```python
from build123d import *

# Parameters (mm, degrees)
F0_W          = 11.8681662488
F0_H          = 19.05
F1_DEPTH      = 12.7
F1_DEPTH_BACK = 12.7
F2_DEPTH      = 6.35
F2_DEPTH_BACK = 6.35
F3_DEPTH      = 12.7
F3_DEPTH_BACK = 12.7
F0_H_2        = 6.35
F4_DEPTH      = 12.7
F4_DEPTH_BACK = 12.7
F6_DEPTH      = 12.7


with BuildPart() as f1:
    # F0 (on Front) → F1 (new body, two sides)
    with BuildSketch(Plane.XZ) as f1_sk:
        with Locations((-36.0392803956, -20.5900701019)):
            Rectangle(F0_W, F0_H)
    extrude(amount=F1_DEPTH)
    extrude(f1_sk.sketch, amount=-F1_DEPTH_BACK)

    # F0 (on Front) → F2 (join, two sides)
    with BuildSketch(Plane.XZ) as f2_sk:
        with BuildLine():
            Line((-30.1051972712, -11.0650701019), (-30.1051972712, -30.1150701019))
            Line((-30.1051972712, -30.1150701019), (-16.57336352, -30.1150701019))
            ThreePointArc((-16.57336352, -30.1150701019), (-26.09836352, -20.5900701019), (-16.57336352, -11.0650701019))
            Line((-16.57336352, -11.0650701019), (-30.1051972712, -11.0650701019))
        make_face()
    extrude(amount=F2_DEPTH)
    extrude(f2_sk.sketch, amount=-F2_DEPTH_BACK)

    # F0 (on Front) → F3 (join, two sides)
    with BuildSketch(Plane.XZ) as f3_sk:
        with BuildLine():
            Line((-16.57336352, -26.9400701019), (-16.57336352, -30.1150701019))
            ThreePointArc((-16.57336352, -30.1150701019), (-9.8381714292, -27.3252621927), (-7.04836352, -20.5900701019))
            ThreePointArc((-7.04836352, -20.5900701019), (-9.8381714292, -13.8548780111), (-16.57336352, -11.0650701019))
            Line((-16.57336352, -11.0650701019), (-16.57336352, -14.2400701019))
            ThreePointArc((-16.57336352, -14.2400701019), (-12.0832354595, -16.0999420414), (-10.22336352, -20.5900701019))
            ThreePointArc((-10.22336352, -20.5900701019), (-12.0832354595, -25.0801981625), (-16.57336352, -26.9400701019))
        make_face()
        with BuildLine():
            ThreePointArc((-16.57336352, -11.0650701019), (-26.09836352, -20.5900701019), (-16.57336352, -30.1150701019))
            Line((-16.57336352, -30.1150701019), (-16.57336352, -26.9400701019))
            ThreePointArc((-16.57336352, -26.9400701019), (-22.92336352, -20.5900701019), (-16.57336352, -14.2400701019))
            Line((-16.57336352, -14.2400701019), (-16.57336352, -11.0650701019))
        make_face()
    extrude(amount=F3_DEPTH)
    extrude(f3_sk.sketch, amount=-F3_DEPTH_BACK)

    # F0 (on Front) → F4 (join, two sides)
    with BuildSketch(Plane.XZ) as f4_sk:
        with Locations((-36.0392803956, -7.8900701019)):
            Rectangle(F0_W, F0_H_2)
    extrude(amount=F4_DEPTH)
    extrude(f4_sk.sketch, amount=-F4_DEPTH_BACK)

    # F5 (on face) → F6 (cut)
    with BuildSketch(Plane.YZ.offset(-30.1051972712)):
        Polygon((12.7, -4.7150701019), (6.35, -4.7150701019), (12.7, -11.0650701019), align=None)
        Polygon((-12.7, -11.0650701019), (-6.35, -4.7150701019), (-12.7, -4.7150701019), align=None)
    extrude(amount=-F6_DEPTH, mode=Mode.SUBTRACT)


solid = f1.part
```
Check sheet for the modelled part. Datum: model origin and axes. Units: mm. A direction names the side the tool comes from. Round coordinates to 2 decimals unless told otherwise and drop trailing zeros. Loops run counter-clockwise (first coordinate to the right, second up) from the corner with the lowest first, then second, coordinate; pieces in that order, holes last. Notation, with made-up numbers: (2, -3.75) -> (41, -3.75) arc R33 ccw to (41, 28.25) -> close; hole circle Ø2 at (57, 4). An arc over 180 degrees is marked (long way). Write item = value, one per line. Start each with the question number.
1) Thickness scan on probe 1 along X at (y, z) = (-10.25, -13.5); probe 2 along X at (y, z) = (-7, -15); probe 3 along Z at (x, y) = (-25, 0.5). Record the ranges inside material, lowest first.
2) Release check for a two-part mould opening along X. For faces 1 (the flat face through (-26.4, 6.35, -20.5)), 2 (the flat face through (-41.973, 0, -18)), 3 (the flat face through (-36, -12.7, -20)) record: released by +X, released by -X, zero draft, split by the parting line, or undercut.
3) Gauge pin test, flat ends, axial feed: pin 1 Ø5 at (y, z) = (2.5, -8.5) entering from +X; pin 2 Ø1.5 at (x, y) = (-12.5, 6.5) entering from -Z; pin 3 Ø5 at (x, z) = (-38, -7.5) entering from +Y. Record the tip position at first contact, or that the pin passes through.
4) Sectioned sample at A-A, the plane y = -8. Record the cut outline in (x, z) (3 decimals).
5) Sectioned sample at B-B, the plane x = -19.5. Record the cut outline in (y, z).
6) Sectioned sample at C-C, the plane y = 2.25. Record the cut outline in (x, z) (3 decimals), plus the area to 3 significant figures.
7) Sectioned sample at D-D, the plane z = -28.5. Record the cut outline in (x, y), plus the area to 3 significant figures.
8) Set-up check for faces 4 (the flat face through (-36, 12.7, -20)), 5 (the flat face through (-23, 0, -11.065)), 6 (the flat face through (-30.105, 0, -9)): record each of +Z, -Z, +X, -X, +Y, -Y from which the full face is reachable in a straight line by a thin tool's end or side.
Results are:
q1.probe_1 = -41.97 to -30.11, -22.93 to -10.21
q1.probe_2 = -41.97 to -30.11, -24.29 to -19.59, -13.56 to -8.86
q1.probe_3 = -30.12 to -11.07
q2.face_1 = undercut
q2.face_2 = released by -X
q2.face_3 = zero draft
q3.pin_1 = -30.11
q3.pin_2 = -29.52
q3.pin_3 = 11.63
q4.outline = (-41.973, -30.115) -> (-30.105, -30.115) -> (-30.105, -6.365) -> (-41.973, -6.365) -> close; circle Ø19.05 at (-16.573, -20.59); hole circle Ø12.7 at (-16.573, -20.59)
q5.outline = (-12.7, -29.65) -> (-6.35, -29.65) -> (-6.35, -30.12) -> (6.35, -30.12) -> (6.35, -29.65) -> (12.7, -29.65) -> (12.7, -26.23) -> (-12.7, -26.23) -> close; (-12.7, -14.95) -> (12.7, -14.95) -> (12.7, -11.53) -> (6.35, -11.53) -> (6.35, -11.07) -> (-6.35, -11.07) -> (-6.35, -11.53) -> (-12.7, -11.53) -> close
q6.outline = (-41.973, -30.115) -> (-16.573, -30.115) arc R9.525 ccw to (-16.573, -11.065) -> (-30.105, -11.065) -> (-30.105, -4.715) -> (-41.973, -4.715) -> close; hole circle Ø12.7 at (-16.573, -20.59)
q6.area = 575 mm^2
q7.outline = (-41.97, -12.7) -> (-30.11, -12.7) -> (-30.11, -6.35) -> (-21.88, -6.35) -> (-21.88, -12.7) -> (-11.27, -12.7) -> (-11.27, 12.7) -> (-21.88, 12.7) -> (-21.88, 6.35) -> (-30.11, 6.35) -> (-30.11, 12.7) -> (-41.97, 12.7) -> close
q7.area = 675 mm^2
q8.face_4 = +Z, -Z, +X, -X, +Y
q8.face_5 = +Z, +X, +Y, -Y
q8.face_6 = +Z
